Input: part model. Units: mm. Frame: model coordinates. Face numbers are marked on the shaded views. A direction names the side the tool comes from. Coordinates: 2 decimals unless noted, no trailing zeros. Loops run counter-clockwise (first coordinate to the right, second up) from the corner with the lowest first, then second, coordinate; pieces in that order, holes last.
(1) Section B-B, the plane y = 0. Return loops of the section in (x, z).
(2) Mould query, pull axis Z, two halves, no side actions, for the marked faces 1, 2 and 3. Classes: released by +Z, released by -Z, zero draft, split by the parting line, or undercut.
(3) Section C-C, the plane z = 11. Return loops of the section in (x, y).
(4) Contact query for flat-ended pins moving along their axis: P1, Ø2, axis at x = 5, y = 8, coming from the +Z side; P2, Ø2, axis at y = 4, z = 2.5, coming from the +X side; P3, Ø2.5, axis at x = 0, y = 0, coming from the +Z side; P4, Ø1.8, axis at x = 0, z = 8, coming from the +Y side. Output: stop coordinate, or through.
(5) Section D-D, the plane x = -4. Return loops of the section in (y, z).
(6) Section A-A, the plane x = 0. Return loops of the section in (y, z), then the cut area to 3 significant figures.
(7) Set-up query: the marked faces 4 and 5. Return all of +Z, -Z, +X, -X, +Y, -Y with unobstructed straight access to the full face (end or side cutting, diameter ignored); none if empty.
(8) Line query: L1, parallel to Y at x = 0, z = 4.5; L2, parallel to Z at x = -3.5, y = -10; L3, parallel to Z at x = 0, y = -3.95. Output: solid intervals per line, ascending.
```python
from build123d import *

# Parameters (mm, degrees)
SKETCH2_R               = 11
SKETCH2_R_2             = 2
SKETCH2_R_3             = 1.244152151
BOSS_EXTRUDE1_DEPTH     = 3
SKETCH3_R               = 5
SKETCH3_R_2             = 2
BOSS_EXTRUDE3_DEPTH     = 10
CUT_EXTRUDE2_REACH      = 22.273
CUT_EXTRUDE2_END_RADIUS = 5
SKETCH6_R               = 1.5


with BuildPart() as part:
    # Sketch2 → Boss-Extrude1 (new body)
    with BuildSketch(Plane.XY):
        Circle(SKETCH2_R)
        Circle(SKETCH2_R_2, mode=Mode.SUBTRACT)
        with Locations((-5.656854249, 5.656854249)):
            Circle(SKETCH2_R_3, mode=Mode.SUBTRACT)
        with Locations((5.656854249, 5.656854249)):
            Circle(SKETCH2_R_3, mode=Mode.SUBTRACT)
        with Locations((5.656854249, -5.656854249)):
            Circle(SKETCH2_R_3, mode=Mode.SUBTRACT)
        with Locations((-5.656854249, -5.656854249)):
            Circle(SKETCH2_R_3, mode=Mode.SUBTRACT)
    extrude(amount=BOSS_EXTRUDE1_DEPTH)

    # Sketch3 → Boss-Extrude3 (add)
    with BuildSketch(Plane.XY.offset(3)):
        Circle(SKETCH3_R)
        Circle(SKETCH3_R_2, mode=Mode.SUBTRACT)
    extrude(amount=BOSS_EXTRUDE3_DEPTH)

    # Cut-Extrude2: up to this cylinder (the profile starts inside it)
    cut_extrude2_end = Plane(origin=(0, 0, 8), z_dir=(0, 0, -1)) * Cylinder(CUT_EXTRUDE2_END_RADIUS, 55.546, mode=Mode.PRIVATE)
    # Sketch6 → Cut-Extrude2 (cut, up to the surface)
    with BuildSketch(Plane(origin=(0, 0, 0), x_dir=(1, 0, 0), z_dir=(0, 1, 0)), mode=Mode.PRIVATE) as cut_extrude2_sk1:
        with Locations(Location((0, -8, 0), (0, 0, 270))):
            Circle(SKETCH6_R)
    cut_extrude2_tool1 = extrude(cut_extrude2_sk1.sketch, amount=-CUT_EXTRUDE2_REACH, mode=Mode.PRIVATE) & cut_extrude2_end
    add(cut_extrude2_tool1.solids().sort_by_distance((0, 0, 8))[0], mode=Mode.SUBTRACT)


solid = part.part
```
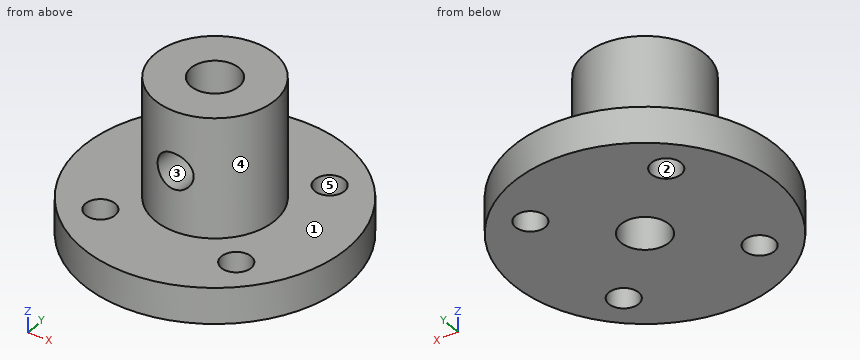
Report:
1. outline: (-11, 0) - (-2, 0) - (-2, 13) - (-5, 13) - (-5, 3) - (-11, 3) - close; (2, 0) - (11, 0) - (11, 3) - (5, 3) - (5, 13) - (2, 13) - close
2. face 1: released by +Z
2. face 2: zero draft
2. face 3: undercut
3. outline: circle Ø10 at (0, 0); hole circle Ø4 at (0, 0)
4. P1: stops at z = 3
4. P2: stops at x = 10.58
4. P3: passes through
4. P4: stops at y = 5
5. outline: (-10.25, 0) - (10.25, 0) - (10.25, 3) - (3, 3) - (3, 13) - (-3, 13) - (-3, 3) - (-10.25, 3) - close
6. outline: (-11, 0) - (-2, 0) - (-2, 6.5) - (-5, 6.5) - (-5, 3) - (-11, 3) - close; (-5, 9.5) - (-2, 9.5) - (-2, 13) - (-5, 13) - close; (2, 0) - (11, 0) - (11, 3) - (5, 3) - (5, 13) - (2, 13) - close
6. area: 105 mm2
7. face 4: +Z
7. face 5: +Z, -Z
8. L1: y = -5 to -2, 2 to 5
8. L2: z = 0 to 3
8. L3: z = 0 to 6.5, 9.5 to 13
